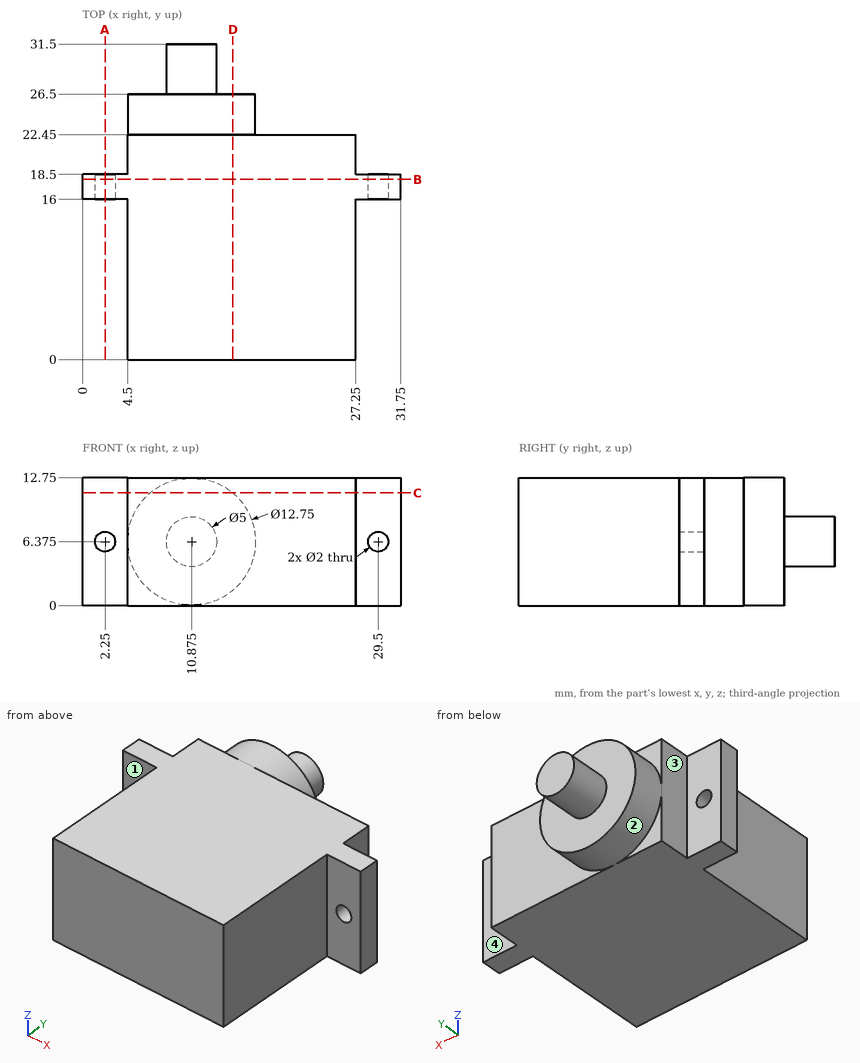
Geometry check sheet. Reference: drawing and pictorial views, mm from the part's lowest x, y, z. A direction names the side the tool comes from. Coordinates: 2 decimals unless noted, no trailing zeros. Loops run counter-clockwise (first coordinate to the right, second up) from the corner with the lowest first, then second, coordinate; pieces in that order, holes last. Notation, with made-up numbers: (13, -8) - (66, -8) arc R20 ccw to (66, 23) - close; hole circle Ø9 at (17.25, 50.25). An arc over 180 degrees is marked (long way). Return JSON: item names as keys, results as strings.
1. Tool access check on the marked faces 1, 2, 3 and 4. Record the directions out of +Z, -Z, +X, -X, +Y, -Y that give a thin tool (end or side, any length) a straight path to the whole face; none if there is none.
Established:
{"face 1": "+Z, -Z, -X, -Y", "face 2": "+Y", "face 3": "+Z, -Z, -X, +Y", "face 4": "+Z, -Z, +X, +Y"}
2. Section check B-B, the plane y = 18. Record the boundary of the cut face in (x, z) (3 decimals), then the cut area to 3 significant figures.
Established:
{"outline": "(0, 0) - (31.75, 0) - (31.75, 12.75) - (0, 12.75) - close; hole circle Ø2 at (2.25, 6.375); hole circle Ø2 at (29.5, 6.375)", "area": "399 mm2"}
3. Thickness scan on L1, parallel to Z at x = 2.25, y = 17.6 (3 decimals); L2, parallel to X at y = 10, z = 6.75; L3, parallel to Y at x = 19, z = 1.25. Record the ranges inside material, lowest first.
Established:
{"L1": "z = 0 to 5.375, 7.375 to 12.75", "L2": "x = 4.5 to 27.25", "L3": "y = 0 to 22.45"}
4. Go/stop test with flat-tipped pins: pin 1 (5 mm diameter, centred on x = 6.5, z = 3, fed in from +Y); pin 2 (1.4 mm diameter, centred on x = 2, z = 5, fed in from -Y); pin 3 (5 mm diameter, centred on x = 28.5, z = 8.5, fed in from -Y); pin 4 (2 mm diameter, centred on x = 30, z = 8.5, fed in from +Y). Record where each tip stops, or that it passes through.
Established:
{"pin 1": "stops at y = 26.5", "pin 2": "stops at y = 16", "pin 3": "stops at y = 0", "pin 4": "stops at y = 18.5"}
5. Section check D-D, the plane x = 15. Record the boundary of the cut face in (y, z), then the cut area to 3 significant figures.
Established:
{"outline": "(0, 0) - (22.45, 0) - (22.45, 1.51) - (26.5, 1.51) - (26.5, 11.24) - (22.45, 11.24) - (22.45, 12.75) - (0, 12.75) - close", "area": "326 mm2"}
6. Section check A-A, the plane x = 2.25. Record the boundary of the cut face in (y, z) (3 decimals), then the cut area to 3 significant figures.
Established:
{"outline": "(16, 0) - (18.5, 0) - (18.5, 5.375) - (16, 5.375) - close; (16, 7.375) - (18.5, 7.375) - (18.5, 12.75) - (16, 12.75) - close", "area": "26.9 mm2"}
7. Section check C-C, the plane z = 11.25. Record the boundary of the cut face in (x, y).
Established:
{"outline": "(0, 16) - (4.5, 16) - (4.5, 0) - (27.25, 0) - (27.25, 16) - (31.75, 16) - (31.75, 18.5) - (27.25, 18.5) - (27.25, 22.45) - (14.98, 22.45) - (14.98, 26.5) - (6.77, 26.5) - (6.77, 22.45) - (4.5, 22.45) - (4.5, 18.5) - (0, 18.5) - close"}
